Here's the drawing with two shaded views (mm, measured from the low corner). I have some questions. Round coordinates to 2 decimals unless told otherwise and drop trailing zeros. Loops run counter-clockwise (first coordinate to the right, second up) from the corner with the lowest first, then second, coordinate; pieces in that order, holes last.
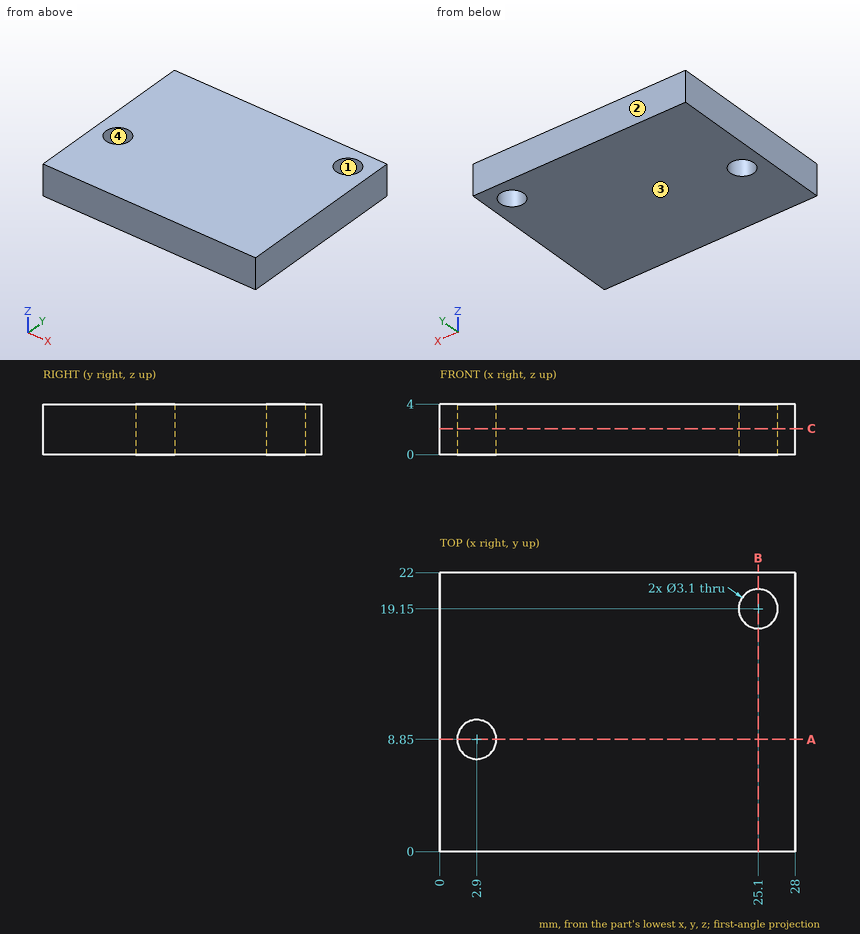
(1) If we section it at A-A, the plane y = 8.85: List the corners of the cut face in (x, z) for me, then the cut area to 3 significant figures.
Worked answers:
outline: (0, 0) - (1.35, 0) - (1.35, 4) - (0, 4) - close; (4.45, 0) - (28, 0) - (28, 4) - (4.45, 4) - close
area: 99.6 mm2
(2) If I drill on line 1 (Y direction, x = 2.9, z = 2.2); line 2 (X direction, y = 18.5, z = 3.8); line 3 (Y direction, x = 2.5, z = 0.2), over which ranges is the centre line in solid material (lowest first)?
Worked answers:
line 1: y = 0 to 7.3, 10.4 to 22
line 2: x = 0 to 23.69, 26.51 to 28
line 3: y = 0 to 7.35, 10.35 to 22
(3) If we section it at B-B, the plane x = 25.1: List the corners of the cut face in (y, z) for me, then the cut area to 3 significant figures.
Worked answers:
outline: (0, 0) - (17.6, 0) - (17.6, 4) - (0, 4) - close; (20.7, 0) - (22, 0) - (22, 4) - (20.7, 4) - close
area: 75.6 mm2
(4) If we mould it in two halves opening along Y, with no side actions, what happens to the marked faces 1, 2, 3 and 4? For each: released by +Y, released by -Y, zero draft, split by the parting line, or undercut.
Worked answers:
face 1: undercut
face 2: released by +Y
face 3: zero draft
face 4: undercut
(5) If we section it at C-C, the plane z = 2.05: List the corners of the cut face in (x, y) for me, then the cut area to 3 significant figures.
Worked answers:
outline: (0, 0) - (28, 0) - (28, 22) - (0, 22) - close; hole circle Ø3.1 at (2.9, 8.85); hole circle Ø3.1 at (25.1, 19.15)
area: 601 mm2
